Job drawing, mm, ordinate dimensions from the low corner. One solid piece. A direction names the side the tool comes from. Give positions to 0.01 mm unless a question says otherwise; leave off trailing zeros. Loops run counter-clockwise (first coordinate to the right, second up) from the corner with the lowest first, then second, coordinate; pieces in that order, holes last. Notation, with made-up numbers: (56, 53) -> (96, 53) arc R25 cw to (96, 77) -> close; hole circle Ø11 at (-30.75, 24). An arc over 180 degrees is marked (long way). Use one line per item in the form item = value.
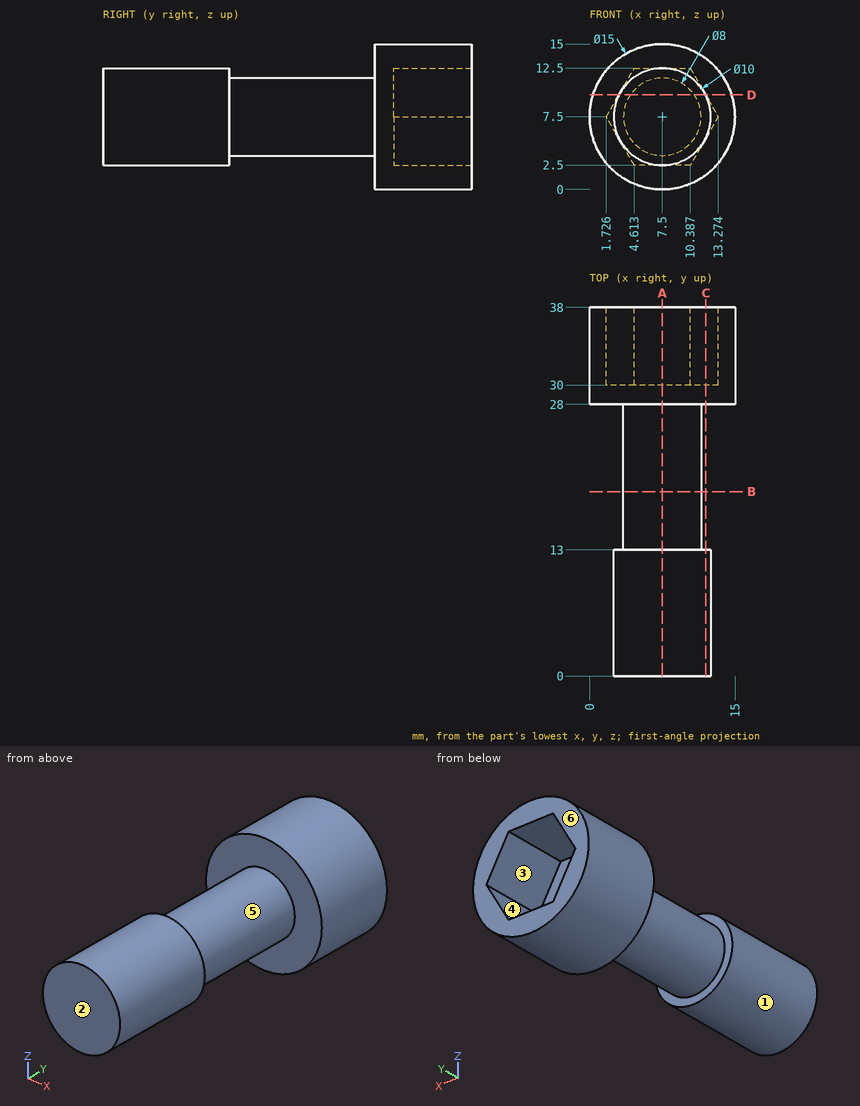
1. Cut at A-A, the plane x = 7.5. Write the cut outline in (y, z), then the cut area to 3 significant figures.
Result sheet:
outline = (0, 2.5) -> (13, 2.5) -> (13, 3.5) -> (28, 3.5) -> (28, 0) -> (38, 0) -> (38, 2.5) -> (30, 2.5) -> (30, 12.5) -> (38, 12.5) -> (38, 15) -> (28, 15) -> (28, 11.5) -> (13, 11.5) -> (13, 12.5) -> (0, 12.5) -> close
area = 320 mm^2
2. Tool access for the marked faces 4, 5 and 6: list every direction of +Z, -Z, +X, -X, +Y, -Y with a clear straight run to the whole face (end or side of a thin tool).
Result sheet:
face_4 = +Y
face_5 = none
face_6 = +Z, -Z, +X, -X, +Y
3. Mould opens along Z. For the marked faces 1, 2 and 3 say: pulls with the +Z half, pulls with the -Z half, needs draft (parallel to the pull), parting line crosses it, or undercut.
Result sheet:
face_1 = parting line crosses it
face_2 = needs draft
face_3 = undercut
4. Cut at C-C, the plane x = 12. Write the cut outline in (y, z) (1 decimal), then the cut area to 3 significant figures.
Result sheet:
outline = (0, 5.3) -> (13, 5.3) -> (13, 9.7) -> (0, 9.7) -> close; (28, 1.5) -> (38, 1.5) -> (38, 5.3) -> (30, 5.3) -> (30, 9.7) -> (38, 9.7) -> (38, 13.5) -> (28, 13.5) -> close
area = 141 mm^2
5. Cut at B-B, the plane y = 19. Write the cut outline in (x, z).
Result sheet:
outline = circle Ø8 at (7.5, 7.5)
6. Cut at D-D, the plane z = 9.75. Write the cut outline in (x, y) (1 decimal), then the cut area to 3 significant figures.
Result sheet:
outline = (0.3, 28) -> (4.2, 28) -> (4.2, 13) -> (3, 13) -> (3, 0) -> (12, 0) -> (12, 13) -> (10.8, 13) -> (10.8, 28) -> (14.7, 28) -> (14.7, 38) -> (12, 38) -> (12, 30) -> (3, 30) -> (3, 38) -> (0.3, 38) -> close
area = 287 mm^2
7. Drill centre lines: line 1 (Y direction, x = 3.5, z = 10.25); line 2 (Z direction, x = 10, y = 34.5); line 3 (Y direction, x = 7.25, z = 7). Where is each one in solid material? Low to high.
Result sheet:
line_1 = 0 to 13, 28 to 30
line_2 = 0.43 to 2.5, 12.5 to 14.57
line_3 = 0 to 30
8. Drop flat-ended pins along their axis: P1, Ø3, axis at x = 3, y = 33, coming from the -Z side (1 decimal); P2, Ø5, axis at x = 9.5, y = 24.5, coming from the -Z side; P3, Ø6, axis at y = 30, z = 4.5, coming from the +X side; P4, Ø4, axis at y = 15.5, z = 4, coming from the -X side. Give the stop position or say it passes through.
Result sheet:
P1 = 0.6
P2 = 3.5
P3 = 15
P4 = 3.79
